from build123d import *

# Parameters (mm, degrees)
SKETCH2_R           = 1.6
SKETCH2_R_2         = 2.1
BOSS_EXTRUDE1_DEPTH = 3.175


with BuildPart() as part:
    # Sketch2 → Boss-Extrude1 (new body)
    with BuildSketch(Plane(origin=(0, 0, 0), x_dir=(0, 0, -1), z_dir=(1, 0, 0))):
        with BuildLine():
            Line((-16, 5), (-16, -5))
            ThreePointArc((-16, -5), (0, -21), (16, -5))
            Line((16, -5), (16, 5))
            ThreePointArc((16, 5), (0, 21), (-16, 5))
        make_face()
        with Locations((-8, -13)):
            Circle(SKETCH2_R, mode=Mode.SUBTRACT)
        with Locations((0, -6.313708499)):
            Circle(SKETCH2_R_2, mode=Mode.SUBTRACT)
        with Locations((8, -13)):
            Circle(SKETCH2_R, mode=Mode.SUBTRACT)
        with Locations((-11.313708499, 5)):
            Circle(SKETCH2_R_2, mode=Mode.SUBTRACT)
        with Locations((0, 16.313708499)):
            Circle(SKETCH2_R_2, mode=Mode.SUBTRACT)
        with Locations((11.313708499, 5)):
            Circle(SKETCH2_R_2, mode=Mode.SUBTRACT)
    extrude(amount=BOSS_EXTRUDE1_DEPTH)


solid = part.part
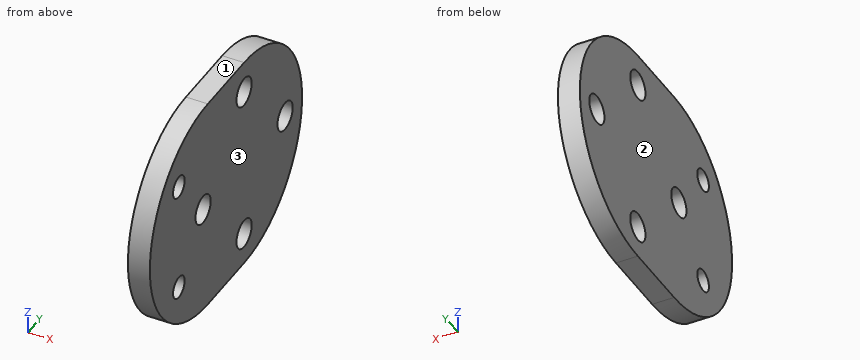
Design review of the part built by this model. Coordinates are the model's own, in mm. Face numbers are marked on the shaded views. Round coordinates to 2 decimals unless told otherwise and drop trailing zeros. Write each loop counter-clockwise with the first axis right and the second up, starting at its lowest first coordinate (ties: lowest second). Pieces come first, ordered by that corner, then holes. Notation, with made-up numbers: (-14, 0) - (12, 0) arc R22 ccw to (12, 6) - close; hole circle Ø5 at (-14, 85.5). An arc over 180 degrees is marked (long way). Return JSON: item names as keys, results as strings. Group by question number.
Item 1: We need section A-A on z = 0. Write out the cut boundary in (x, y) (3 decimals).
Item 2: The part is to be moulded in two halves that separate along X. For the marked faces 1, 2 and 3, say which applies: pulls with the +X half, pulls with the -X half, needs draft (parallel to the pull), parting line crosses it, or undercut.
Item 3: We need section B-B on z = 10.5. Write out the cut boundary in (x, y) (3 decimals), and give its area (3 significant figures).
Item 4: Insertion check: P1, Ø4, axis at y = 5, z = 11.31, coming from the +X side; P2, Ø1, axis at x = 2.5, y = -10, coming from the +Z side. Each pin has a flat end and moves straight along its axis. Give the tip position at first contact, or say it passes through.
Item 5: For probe 1 along Y at (x, z) = (1.45, 0); probe 2 along Y at (x, z) = (0.3, -1); probe 3 along Z at (x, y) = (3, 17.5), list the stretches that pass through material, from the lowest coordinate up. Write a range as [from, to].
Item 6: We need section D-D on x = 1.6. Write out the cut boundary in (y, z), and give its area (3 significant figures).
Item 7: We need section C-C on y = -13. Write out the cut boundary in (x, z) (3 decimals).
Model answer:
{
 "1": {"outline": "(0, -21) - (3.175, -21) - (3.175, -8.414) - (0, -8.414) - close; (0, -4.214) - (3.175, -4.214) - (3.175, 14.214) - (0, 14.214) - close; (0, 18.414) - (3.175, 18.414) - (3.175, 21) - (0, 21) - close"},
 "2": {"face 1": "needs draft", "face 2": "pulls with the -X half", "face 3": "pulls with the +X half"},
 "3": {"outline": "(0, -17.073) - (3.175, -17.073) - (3.175, 3.064) - (0, 3.064) - close; (0, 6.936) - (3.175, 6.936) - (3.175, 17.073) - (0, 17.073) - close", "area": "96.1 mm²"},
 "4": {"P1": "passes through", "P2": "stops at z = 15.35"},
 "5": {"probe 1": "y = [-21, -8.41], [-4.21, 14.21], [18.41, 21]", "probe 2": "y = [-20.97, -8.16], [-4.47, 14.47], [18.16, 20.97]", "probe 3": "z = [-9.99, -1.73], [1.73, 9.99]"},
 "6": {"outline": "(-5, -16) - (5, -16) arc R16 ccw to (5, 16) - (-5, 16) arc R16 ccw to start; hole circle Ø3.2 at (-13, -8); hole circle Ø3.2 at (-13, 8); hole circle Ø4.2 at (-6.31, 0); hole circle Ø4.2 at (5, -11.31); hole circle Ø4.2 at (5, 11.31); hole circle Ø4.2 at (16.31, 0)", "area": "1,050 mm²"},
 "7": {"outline": "(0, -13.856) - (3.175, -13.856) - (3.175, -9.6) - (0, -9.6) - close; (0, -6.4) - (3.175, -6.4) - (3.175, 6.4) - (0, 6.4) - close; (0, 9.6) - (3.175, 9.6) - (3.175, 13.856) - (0, 13.856) - close"}
}
